from build123d import *

# Parameters (mm, degrees)
ESQUISSE1_R             = 10
BOSS_EXTRU_1_DEPTH      = 4
ESQUISSE2_R             = 3.5
BOSS_EXTRU_2_DEPTH      = 14.13
BOSS_EXTRU_3_DEPTH      = 20
ESQUISSE4_R             = 1.25
ENL_V_MAT_EXTRU_1_DEPTH = 100
ESQUISSE5_R             = 0.75
ENL_V_MAT_EXTRU_2_DEPTH = 14
ESQUISSE6_R             = 2.127089322
ENL_V_MAT_EXTRU_3_DEPTH = 1.5
ESQUISSE7_R             = 4.3
ESQUISSE7_R_2           = 3.5
BOSS_EXTRU_4_DEPTH      = 9.13


with BuildPart() as part:
    # Esquisse1 → Boss.-Extru.1 (new body)
    with BuildSketch(Plane.XY):
        Circle(ESQUISSE1_R)
    extrude(amount=BOSS_EXTRU_1_DEPTH)

    # Esquisse2 → Boss.-Extru.2 (add)
    with BuildSketch(Plane.XY.offset(4)):
        Circle(ESQUISSE2_R)
    extrude(amount=BOSS_EXTRU_2_DEPTH)

    # Esquisse3 → Boss.-Extru.3 (add)
    with BuildSketch(Plane.XY.offset(18.13)):
        Polygon((-1.190476286, 3.29131679), (-3.445602095, 0.614675689), (-2.255125809, -2.676641101), (1.190476286, -3.29131679), (3.445602095, -0.614675689), (2.255125809, 2.676641101), align=None)
    extrude(amount=BOSS_EXTRU_3_DEPTH)

    # Esquisse4 → Enlèv. mat.-Extru.1 (cut)
    with BuildSketch(Plane(origin=(0, 0, 0), x_dir=(-1, 0, 0), z_dir=(0, 0, -1))):
        with Locations((2.241387648, 6.631453944)):
            Circle(ESQUISSE4_R)
        with Locations((-6.631453944, 2.241387648)):
            Circle(ESQUISSE4_R)
        with Locations((6.631453944, -2.241387648)):
            Circle(ESQUISSE4_R)
        with Locations((-2.241387648, -6.631453944)):
            Circle(ESQUISSE4_R)
    extrude(amount=-ENL_V_MAT_EXTRU_1_DEPTH, mode=Mode.SUBTRACT)

    # Esquisse5 → Enlèv. mat.-Extru.2 (cut)
    with BuildSketch(Plane(origin=(0.532324762, 2.983978946, 0), x_dir=(0.984457741, -0.175621625, 0), z_dir=(0.175621625, 0.984457741, 0))):
        with Locations((0, -28.127949192)):
            Circle(ESQUISSE5_R)
    extrude(amount=-ENL_V_MAT_EXTRU_2_DEPTH, mode=Mode.SUBTRACT)

    # Esquisse6 → Enlèv. mat.-Extru.3 (cut)
    with BuildSketch(Plane(origin=(0, 0, 0), x_dir=(-1, 0, 0), z_dir=(0, 0, -1))):
        Circle(ESQUISSE6_R)
    extrude(amount=-ENL_V_MAT_EXTRU_3_DEPTH, mode=Mode.SUBTRACT)

    # Esquisse7 → Boss.-Extru.4 (add)
    with BuildSketch(Plane.XY.offset(4)):
        Circle(ESQUISSE7_R)
        Circle(ESQUISSE7_R_2, mode=Mode.SUBTRACT)
    extrude(amount=BOSS_EXTRU_4_DEPTH)


solid = part.part
The model under review builds one solid part; all positions refer to its coordinate system, in mm. A direction names the side the tool comes from. Round coordinates to 2 decimals unless told otherwise and drop trailing zeros. Order: outer loops, then holes, each group sorted by start corner. A loop starts at its lowest first (then second) coordinate and runs counter-clockwise, first axis right, second up. Notation, with made-up numbers: (70.5, 86) -> (87.5, 86) arc R12 ccw to (87.5, 101) -> close; hole circle Ø3 at (14.5, 75.25). An arc over 180 degrees is marked (long way). Use CSV: the item, a comma, the result in double quotes. Start each with the question number.
(1) Insertion check: pin 1 (3 mm diameter, centred on x = 2.24, y = -6.63, fed in from +Z); pin 2 (5 mm diameter, centred on x = -4, z = 30, fed in from +Y); pin 3 (8 mm diameter, centred on x = 6, z = 17, fed in from -Y). Each pin has a flat end and moves straight along its axis. Give the tip position at first contact, or say it passes through.
(2) Consider section B-B on z = 26. Write out the cut boundary in (x, y).
(3) Consider section D-D on z = 17. Write out the cut boundary in (x, y).
(4) Mouldability with a two-part tool opening along X and no side actions: class faces 1 (the face through (-2.17, -9.76, 1.97)), 2 (the face through (2.302, -1.972, 27.99)), 3 (the face through (-7.824, -1.866, 1.972)), 4 (the face through (-0.6, -3.2, 18.13)) as pulls with the +X half, pulls with the -X half, needs draft (parallel to the pull), parting line crosses it, or undercut.
(5) Tool access review of faces 5 (the face through (3.233, -1.341, 15.595)), 6 (the face through (2.86, 1.01, 27.99)), 7 (the face through (2.5, -2.1, 18.13)): name each direction out of +Z, -Z, +X, -X, +Y, -Y from which nothing blocks a thin tool from reaching the whole face with its end or side.
(6) Consider section A-A on y = -6.25. Write out the cut boundary in (x, z), and give its area (3 significant figures).
(7) Wall thickness on probe 1 along Z at (x, y) = (-7.75, 6); probe 2 along Z at (x, y) = (2, 3.5); probe 3 along X at (y, z) = (-2.5, 6): over which ranges is each line inside the solid? List them lowest first. Write a range as from..to.
(8) Consider section C-C on y = 6. Write out the cut boundary in (x, z), and give its area (3 significant figures).
Responses:
1,pin 1,"z = 4"
1,pin 2,"y = 2.92"
1,pin 3,"y = -2.87"
2,outline,"(-3.45, 0.61) -> (-2.26, -2.68) -> (1.19, -3.29) -> (3.45, -0.61) -> (2.26, 2.68) -> (-1.19, 3.29) -> close"
3,outline,"circle Ø7 at (0, 0)"
4,face 1,"parting line crosses it"
4,face 2,"pulls with the +X half"
4,face 3,"undercut"
4,face 4,"needs draft"
5,face 5,"+Z"
5,face 6,"+Z, +X, +Y"
5,face 7,"+Z, +X, -Y"
6,outline,"(-7.81, 0) -> (1.05, 0) -> (1.05, 4) -> (-7.81, 4) -> close; (3.43, 0) -> (7.81, 0) -> (7.81, 4) -> (3.43, 4) -> close"
6,area,"52.9 mm²"
7,probe 1,"0..4"
7,probe 2,"0..13.13"
7,probe 3,"-3.5..3.5"
8,outline,"(-8, 0) -> (-3.32, 0) -> (-3.32, 4) -> (-8, 4) -> close; (-1.16, 0) -> (8, 0) -> (8, 4) -> (-1.16, 4) -> close"
8,area,"55.4 mm²"
